The listing builds one solid part. Answer for the finished solid, in the listing's coordinates (mm). Face numbers are marked on the shaded views. Give positions to 0.01 mm unless a question says otherwise; leave off trailing zeros. Order: outer loops, then holes, each group sorted by start corner. A loop starts at its lowest first (then second) coordinate and runs counter-clockwise, first axis right, second up. Notation, with made-up numbers: (37, -40) - (57, -40) arc R26 ccw to (57, -11) - close; hole circle Ø3 at (84.25, -36). An arc over 180 degrees is marked (long way). Answer in a Markdown table with one row per item.
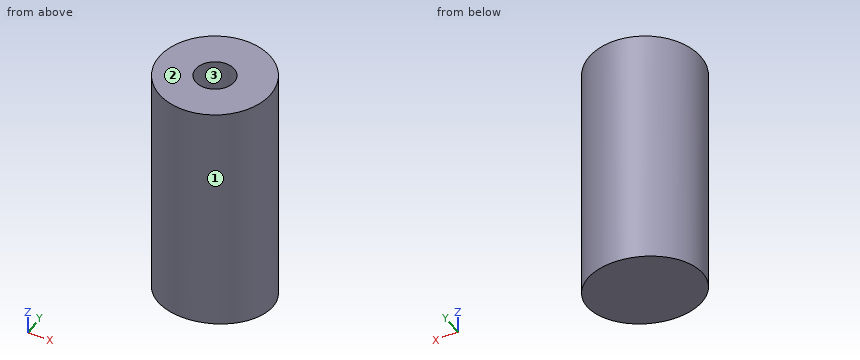
Autodesk Inventor part; units mm, degrees
ref_plane "YZ Plane" through (0, 0, 0) normal (1, 0, 0) x (0, 1, 0)
ref_plane "XZ Plane" through (0, 0, 0) normal (0, 1, 0) x (-1, 0, 0)
ref_plane "XY Plane" through (0, 0, 0) normal (0, 0, 1) x (1, 0, 0)
sketch "Sketch1" plane through (0, 0, 0) normal (0, 0, 1) x (1, 0, 0)
  circle A0 centre (0, 0) radius 7.2
  dimension "d0" = 14.4
extrude "Extrusion1" add sketch "Sketch1" along normal blind 32
sketch "Sketch2" plane through (0, 0, 32) normal (0, 0, 1) x (1, 0, 0)
  circle A0 centre (0, 0) radius 2.5
  dimension "d3" = 5
extrude "Extrusion2" cut sketch "Sketch2" against normal blind 10
sketch "Sketch3" plane through (0, 0, 0) normal (0, 0, 1) x (1, 0, 0)
  circle A0 centre (0, 0) radius 7.2
  line L0 (11.2434, 7.2) -> (-13.4853, 7.2) construction
ref_plane "Work Plane1" through (11.2434, 7.2, 0) normal (0, -0.1297, -0.9916) x (-1, 0, 0)
sketch "Sketch4" plane through (11.2434, 7.2, 0) normal (0, -0.1297, -0.9916) x (-1, 0, 0)
  line L0 (30.8181, -24.4459) -> (-8.3313, -24.4459)
  line L1 (-8.3313, -24.4459) -> (-8.3313, 10.1675)
  line L2 (-8.3313, 10.1675) -> (30.8181, 10.1675)
  line L3 (30.8181, 10.1675) -> (30.8181, -24.4459)
  line L4 (30.8181, -24.4459) -> (-8.3313, 10.1675) construction
  line L5 (-8.3313, -24.4459) -> (30.8181, 10.1675) construction
  point P0 (11.2434, -7.1392)
extrude "Extrusion3" cut sketch "Sketch4" along normal blind 10
properties part number "HoleFill1"
Item 1: Find section A-A on x = 0. Write down the section's boundary in (y, z), then the cut area to 3 significant figures.
Answer block:
| item | result |
|---|---|
| outline | (-7.2, 1.89) - (7.2, 0) - (7.2, 32) - (2.5, 32) - (2.5, 22) - (-2.5, 22) - (-2.5, 32) - (-7.2, 32) - close |
| area | 397 mm² |
Item 2: Determine the mould class of the marked faces 1, 2 and 3 for opening direction Y: pulls with the +Y half, pulls with the -Y half, needs draft (parallel to the pull), parting line crosses it, or undercut.
Answer block:
| item | result |
|---|---|
| face 1 | parting line crosses it |
| face 2 | needs draft |
| face 3 | undercut |
Item 3: Each of these flat-tipped pins is pushed along its axis until it touches: P1, Ø4, axis at x = 0, y = 0, coming from the +Z side; P2, Ø4, axis at x = -3, z = 4, coming from the +Y side; P3, Ø1, axis at x = -5, z = 20, coming from the +Y side. Where does it stop, or does it pass through?
Answer block:
| item | result |
|---|---|
| P1 | z = 22 |
| P2 | y = 7.13 |
| P3 | y = 5.62 |
Item 4: Find section D-D on y = -4.75. Write down the section's boundary in (x, z), then the cut area to 3 significant figures.
Answer block:
| item | result |
|---|---|
| outline | (-5.41, 1.57) - (5.41, 1.57) - (5.41, 32) - (-5.41, 32) - close |
| area | 329 mm² |
Item 5: Find section C-C on z = 13.5. Write down the section's boundary in (x, y).
Answer block:
| item | result |
|---|---|
| outline | circle Ø14.4 at (0, 0) |
Item 6: Find section B-B on y = 0. Write down the section's boundary in (x, z), then the cut area to 3 significant figures.
Answer block:
| item | result |
|---|---|
| outline | (-7.2, 0.94) - (7.2, 0.94) - (7.2, 32) - (2.5, 32) - (2.5, 22) - (-2.5, 22) - (-2.5, 32) - (-7.2, 32) - close |
| area | 397 mm² |
Item 7: Consider line 1 (Y direction, x = 0, z = 26.25); line 2 (Y direction, x = 1, z = 23); line 3 (X direction, y = 3.5, z = 12.5). Determine where each line is inside the solid, lowest interval first.
Answer block:
| item | result |
|---|---|
| line 1 | -7.2 to -2.5, 2.5 to 7.2 |
| line 2 | -7.13 to -2.29, 2.29 to 7.13 |
| line 3 | -6.29 to 6.29 |
